Study the drawing (mm; zero at the part's minimum x, y, z) and answer. Coordinates: 2 decimals unless noted, no trailing zeros. Order: outer loops, then holes, each group sorted by start corner. A loop starts at its lowest first (then second) coordinate and runs counter-clockwise, first axis right, second up.
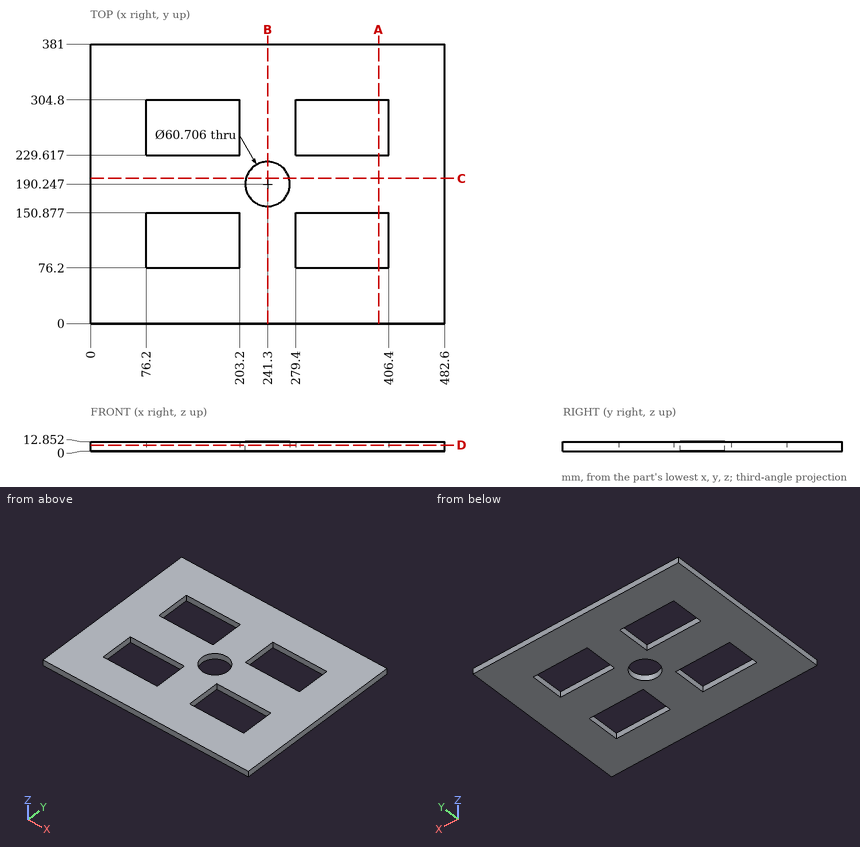
1) A cutting plane is placed at B-B, the plane x = 241.3. Determine the outline of the cut face in (y, z).
A:
outline: (0, 0) - (159.89, 0) - (159.89, 12.85) - (0, 12.85) - close; (220.6, 0) - (381, 0) - (381, 12.85) - (220.6, 12.85) - close
2) A cutting plane is placed at D-D, the plane z = 8.25. Determine the outline of the cut face in (x, y).
A:
outline: (0, 0) - (482.6, 0) - (482.6, 381) - (0, 381) - close; hole (76.2, 76.2) - (203.2, 76.2) - (203.2, 150.88) - (76.2, 150.88) - close; hole (76.2, 229.62) - (203.2, 229.62) - (203.2, 304.8) - (76.2, 304.8) - close; hole circle Ø60.71 at (241.3, 190.25); hole (279.4, 76.2) - (406.4, 76.2) - (406.4, 150.88) - (279.4, 150.88) - close; hole (279.4, 229.62) - (406.4, 229.62) - (406.4, 304.8) - (279.4, 304.8) - close
3) Straight lines are drawn through the part: line 1 (Y direction, x = 167, z = 0.5); line 2 (X direction, y = 288, z = 5.25); line 3 (Y direction, x = 241.3, z = 9.25). For each, find the intervals that lie inside material, in ascending order.
A:
line 1: y = 0 to 76.2, 150.88 to 229.62, 304.8 to 381
line 2: x = 0 to 76.2, 203.2 to 279.4, 406.4 to 482.6
line 3: y = 0 to 159.89, 220.6 to 381
4) A cutting plane is placed at A-A, the plane x = 392.5. Determine the outline of the cut face in (y, z).
A:
outline: (0, 0) - (76.2, 0) - (76.2, 12.85) - (0, 12.85) - close; (150.88, 0) - (229.62, 0) - (229.62, 12.85) - (150.88, 12.85) - close; (304.8, 0) - (381, 0) - (381, 12.85) - (304.8, 12.85) - close
5) A cutting plane is placed at C-C, the plane y = 198. Determine the outline of the cut face in (x, z).
A:
outline: (0, 0) - (211.95, 0) - (211.95, 12.85) - (0, 12.85) - close; (270.65, 0) - (482.6, 0) - (482.6, 12.85) - (270.65, 12.85) - close
